from build123d import *

# Parameters (mm, degrees)
SKETCH_1_R    = 1.6
SKETCH_1_R_2  = 1.1
SKETCH_1_R_3  = 1.65
F_1P5MM_DEPTH = 1.5
SKETCH_2_R    = 1.1
D2P2_DEPTH    = 1.5


with BuildPart() as part:
    # 草图1 → 1p5mm竖向开孔板_上下四孔 (new body)
    with BuildSketch(Plane.XY):
        Polygon((-48.804040507, -9), (48.804040507, -9), (51.804040507, -6), (51.804040507, 47), (48.804040507, 50), (-48.804040507, 50), (-51.804040507, 47), (-51.804040507, -6), align=None)
        with Locations((-45.804040507, -0.5)):
            Circle(SKETCH_1_R, mode=Mode.SUBTRACT)
        with Locations((-45.804040507, 43.5)):
            Circle(SKETCH_1_R, mode=Mode.SUBTRACT)
        with Locations((45.804040507, -0.5)):
            Circle(SKETCH_1_R, mode=Mode.SUBTRACT)
        with Locations((45.804040507, 43.5)):
            Circle(SKETCH_1_R, mode=Mode.SUBTRACT)
        with Locations((-21, 3)):
            Circle(SKETCH_1_R_2, mode=Mode.SUBTRACT)
        with Locations((21, 3)):
            Circle(SKETCH_1_R_2, mode=Mode.SUBTRACT)
        with Locations((-14, 11)):
            Circle(SKETCH_1_R_2, mode=Mode.SUBTRACT)
        with Locations((-14, 39)):
            Circle(SKETCH_1_R_2, mode=Mode.SUBTRACT)
        with Locations((14, 11)):
            Circle(SKETCH_1_R_2, mode=Mode.SUBTRACT)
        with Locations((14, 39)):
            Circle(SKETCH_1_R_2, mode=Mode.SUBTRACT)
        with Locations((-17, 8)):
            Circle(SKETCH_1_R_2, mode=Mode.SUBTRACT)
        with Locations((-17, 42)):
            Circle(SKETCH_1_R_2, mode=Mode.SUBTRACT)
        with Locations((17, 8)):
            Circle(SKETCH_1_R_2, mode=Mode.SUBTRACT)
        with Locations((17, 42)):
            Circle(SKETCH_1_R_2, mode=Mode.SUBTRACT)
        with Locations((-22.5, 25)):
            Circle(SKETCH_1_R_3, mode=Mode.SUBTRACT)
        with Locations((22.5, 25)):
            Circle(SKETCH_1_R_3, mode=Mode.SUBTRACT)
        Polygon((-4, 9.5), (4, 9.5), (7, 12.5), (7, 28.5), (4, 31.5), (-4, 31.5), (-7, 28.5), (-7, 12.5), align=None, mode=Mode.SUBTRACT)
        Polygon((-40, 3.5), (-32, 3.5), (-30, 5.5), (-30, 35.5), (-32, 37.5), (-40, 37.5), (-42, 35.5), (-42, 5.5), align=None, mode=Mode.SUBTRACT)
        Polygon((32, 3.5), (40, 3.5), (42, 5.5), (42, 35.5), (40, 37.5), (32, 37.5), (30, 35.5), (30, 5.5), align=None, mode=Mode.SUBTRACT)
        Polygon((-6, -6.5), (6, -6.5), (8, -4.5), (8, 1.5), (6, 3.5), (-6, 3.5), (-8, 1.5), (-8, -4.5), align=None, mode=Mode.SUBTRACT)
        Polygon((-6, 37.5), (6, 37.5), (8, 39.5), (8, 45.5), (6, 47.5), (-6, 47.5), (-8, 45.5), (-8, 39.5), align=None, mode=Mode.SUBTRACT)
    extrude(amount=F_1P5MM_DEPTH)

    # 草图2 → 上沿电池板钢索孔_D2p2 (cut)
    with BuildSketch(Plane.XY):
        with Locations((-21, 47)):
            Circle(SKETCH_2_R)
        with Locations((21, 47)):
            Circle(SKETCH_2_R)
    extrude(amount=D2P2_DEPTH, mode=Mode.SUBTRACT)


solid = part.part
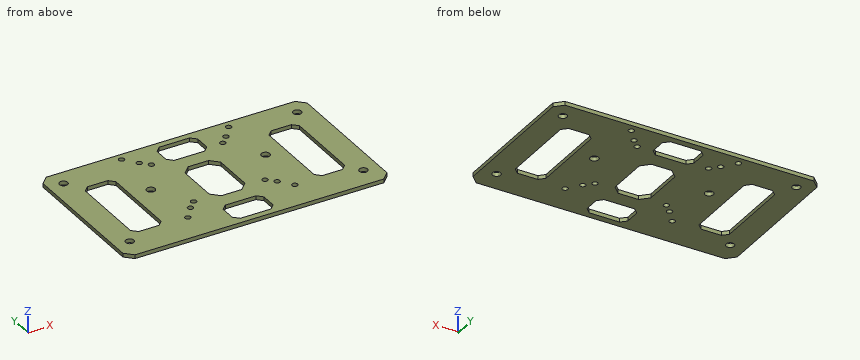
Geometry check sheet. Reference: the model listing, model coordinates, mm. Give positions to 0.01 mm unless a question says otherwise; leave off trailing zeros. Loops run counter-clockwise (first coordinate to the right, second up) from the corner with the lowest first, then second, coordinate; pieces in that order, holes last. Notation, with made-up numbers: (46, 14) -> (101, 14) arc R23 cw to (101, 37) -> close; hole circle Ø1 at (4.25, -23.5). An arc over 180 degrees is marked (long way). Answer in a Markdown table with one row per item. Add a question column.
1) Material ranges on probe 1 along X at (y, z) = (28.5, 0.75); probe 2 along X at (y, z) = (32, 1.45); probe 3 along Y at (x, z) = (-22.5, 0.5), recorded low to high. Write a range as from..to.
2) Cross-section at D-D on y = -0.5. Record the boundary of the cut face in (x, z), and give its area (3 significant figures).
3) Cross-section at C-C on x = 14. Record the boundary of the cut face in (y, z).
4) Gauge pin test, flat ends, axial feed: P1, Ø3, axis at x = -17, y = 42, coming from the -Z side; P2, Ø1.3, axis at x = -17, y = 8, coming from the +Z side. Record the tip position at first contact, or that the pin passes through.
5) Cross-section at A-A on y = 18. Record the boundary of the cut face in (x, z), and give its area (3 significant figures).
6) Cross-section at B-B on x = -41. Record the boundary of the cut face in (y, z), and give its area (3 significant figures).
Outcome:
| question | item | result |
|---|---|---|
| 1 | probe 1 | x = -51.8..-42, -30..-7, 7..30, 42..51.8 |
| 1 | probe 2 | x = -51.8..-42, -30..30, 42..51.8 |
| 1 | probe 3 | y = -9..23.35, 26.65..50 |
| 2 | outline | (-51.8, 0) -> (-47.4, 0) -> (-47.4, 1.5) -> (-51.8, 1.5) -> close; (-44.2, 0) -> (-8, 0) -> (-8, 1.5) -> (-44.2, 1.5) -> close; (8, 0) -> (44.2, 0) -> (44.2, 1.5) -> (8, 1.5) -> close; (47.4, 0) -> (51.8, 0) -> (51.8, 1.5) -> (47.4, 1.5) -> close |
| 2 | area | 122 mm^2 |
| 3 | outline | (-9, 0) -> (9.9, 0) -> (9.9, 1.5) -> (-9, 1.5) -> close; (12.1, 0) -> (37.9, 0) -> (37.9, 1.5) -> (12.1, 1.5) -> close; (40.1, 0) -> (50, 0) -> (50, 1.5) -> (40.1, 1.5) -> close |
| 4 | P1 | stops at z = 0 |
| 4 | P2 | passes through |
| 5 | outline | (-51.8, 0) -> (-42, 0) -> (-42, 1.5) -> (-51.8, 1.5) -> close; (-30, 0) -> (-7, 0) -> (-7, 1.5) -> (-30, 1.5) -> close; (7, 0) -> (30, 0) -> (30, 1.5) -> (7, 1.5) -> close; (42, 0) -> (51.8, 0) -> (51.8, 1.5) -> (42, 1.5) -> close |
| 5 | area | 98.4 mm^2 |
| 6 | outline | (-9, 0) -> (4.5, 0) -> (4.5, 1.5) -> (-9, 1.5) -> close; (36.5, 0) -> (50, 0) -> (50, 1.5) -> (36.5, 1.5) -> close |
| 6 | area | 40.5 mm^2 |
